Verification items for the finished model (mm, model axes). A direction names the side the tool comes from. Coordinates: 2 decimals unless noted, no trailing zeros. Loops run counter-clockwise (first coordinate to the right, second up) from the corner with the lowest first, then second, coordinate; pieces in that order, holes last. Notation, with made-up numbers: (60, -18) - (71, -18) arc R11 cw to (71, 1) - close; hole circle Ø3 at (-19.5, 88). An arc over 180 degrees is marked (long way). Answer as CSV lines item,"result". Start each with the question number.
1. Set-up check for faces 1 (the flat face through (8.5, 2, 0)), 2 (the cylindrical face through (14.725, 10.143, -36.753)), 3 (the flat face through (19.035, 5.65, 42.465)), 4 (the cylindrical face through (8.292, 4.233, -2.999)): record each of +Z, -Z, +X, -X, +Y, -Y from which the full face is reachable in a straight line by a thin tool's end or side.
2. Cross-section at B-B (x = 20). Enter the section's corners in (y, z), plus the area to 3 significant figures.
3. Release check for a two-part mould opening along Y. For faces 5 (the flat face through (8, 20, 1)), 6 (the flat face through (19, 10, 45)), 7 (the flat face through (15, 10, 17)) record: pulls with the +Y half, pulls with the -Y half, needs draft (parallel to the pull), parting line crosses it, or undercut.
4. Gauge pin test, flat ends, axial feed: P1, Ø10.5, axis at y = 10, z = 0, coming from the +X side; P2, Ø1.5, axis at x = 9, y = 13.5, coming from the -Z side; P3, Ø5.5, axis at x = 18, y = 11, coming from the -Z side. Record the tip position at first contact, or that the pin passes through.
5. Cross-section at D-D (x = 1.75). Enter the section's corners in (y, z).
6. Cross-section at A-A (z = 0). Enter the section's corners in (x, y), plus the area to 3 significant figures.
7. Material ranges on line 1 (Y direction, x = 15.15, z = -40); line 2 (Y direction, x = 0.5, z = 0); line 3 (Z direction, x = 18.25, y = 6.75), recorded low to high. Write a range as [from, to].
8. Cross-section at C-C (y = 18). Enter the section's corners in (x, z).
Autodesk Inventor part; units mm, degrees
ref_plane "YZ Plane" through (0, 0, 0) normal (1, 0, 0) x (0, 1, 0)
ref_plane "XZ Plane" through (0, 0, 0) normal (0, 1, 0) x (-1, 0, 0)
ref_plane "XY Plane" through (0, 0, 0) normal (0, 0, 1) x (1, 0, 0)
sketch "Sketch1" plane through (0, 0, 0) normal (0, 1, 0) x (-1, 0, 0)
  line L0 (0, 0) -> (-20, 0)
  line L1 (-20, 0) -> (-20, -40)
  line L2 (-20, -40) -> (0, 0)
  line L3 (-21.5, -50) -> (-18.5, -50)
  line L4 (-18.5, -50) -> (-18.5, -30)
  line L5 (-18.5, -30) -> (-21.5, -30)
  line L6 (-21.5, -30) -> (-21.5, -50)
  line L7 (-21.5, -50) -> (-18.5, -30) construction
  line L8 (-18.5, -50) -> (-21.5, -30) construction
  line L9 (1.5, 10) -> (-1.5, 10)
  line L10 (-1.5, 10) -> (-1.5, -10)
  line L11 (-1.5, -10) -> (1.5, -10)
  line L12 (1.5, -10) -> (1.5, 10)
  line L13 (1.5, 10) -> (-1.5, -10) construction
  line L14 (-1.5, 10) -> (1.5, -10) construction
  line L15 (-1.5, 10) -> (-21.5, -30)
  line L16 (1.5, -10) -> (-18.5, -50)
  line L17 (1.5, -10) -> (1.5, 10)
  line L18 (1.5, -10) -> (1.5, 10)
  line L19 (1.5, 10) -> (-8.5, 10)
  line L20 (-8.5, 10) -> (-8.5, -10)
  line L21 (-8.5, -10) -> (1.5, -10)
  line L22 (1.5, -10) -> (1.5, 10)
  line L23 (0, 0) -> (10, 0)
  line L24 (0, 0) -> (10, 0) construction
  line L25 (-20, 40) -> (0, 0)
  line L26 (-21.5, 50) -> (-18.5, 50)
  line L27 (-18.5, 50) -> (-18.5, 30)
  line L28 (-18.5, 30) -> (-21.5, 30)
  line L29 (-21.5, 30) -> (-21.5, 50)
  line L30 (-1.5, -10) -> (-1.5, 10)
  line L31 (-1.5, 10) -> (1.5, 10)
  line L32 (-1.5, -10) -> (-21.5, 30)
  line L33 (1.5, 10) -> (-18.5, 50)
  line L34 (1.5, 10) -> (1.5, -10)
  point P0 (-7.3579, -1.7157)
  point P1 (-11.5, -10)
  point P2 (-11.5, -10)
  point P3 (-8.5, -4)
  point P4 (-8.5, 4)
  dimension "d0" = 20
  dimension "d1" = 40
  dimension "d2" = 3
  dimension "d3" = 20
  dimension "d4" = 3
  dimension "d5" = 20
  dimension "d31" = 10
  dimension "d32" = 20
  dimension "d42" = 10
  dimension "d43" = 0
extrude "Extrusion1" add sketch "Sketch1" along normal blind 20 contours L2 L10 L0 | L23 L12 L11 L10 L2 | L25 L10 L9 L12 L23 | L0 L10 L25 | L10 L2 L32 L0 | L0 L15 L25 L10 | L10 L32 L2 | L25 L15 L10 | L15 L20 L0 | L32 L20 L19 L25 L15 | L32 L2 L21 L20 L15 | L0 L20 L32 | L32 L21 L2 | L11 L16 L4 L2 L21 | L9 L19 L25 L27 L33 | L15 L25 L19 | L20 L21 L2 L4 L5 L1 L15 | L32 L28 L27 L25 L19 L20 | L3 L6 L5 L1 L2 L4 | L27 L28 L29 L26 | L1 L5 L15 | L2 L1 L5 L4
sketch "Sketch2" plane through (-1.5, 0, -10) normal (-1, 0, 0) x (0, 0, 1)
  circle A0 centre (10, 10) radius 3
  line L0 (0, 0) -> (20, 0)
  line L1 (20, 0) -> (20, 20)
  point P0 (10, 0)
  dimension "d8" = 6
  dimension "d9" = 10
  dimension "d44" = 10
sketch "Sketch3" plane through (21.5, 0, -30) normal (1, 0, 0) x (0, 0, -1)
  circle A0 centre (10, 10) radius 3.25
  line L0 (0, 20) -> (20, 20)
  line L1 (20, 0) -> (20, 20)
  point P0 (-30, 0)
  dimension "d11" = 6.5
  dimension "d12" = 10
  dimension "d13" = 10
extrude "Extrusion2" cut sketch "Sketch2" against normal through all
extrude "Extrusion3" cut sketch "Sketch3" against normal through all
sketch "Sketch4" plane through (21.5, 0, -30) normal (1, 0, 0) x (0, 0, -1)
  circle A0 centre (10, 10) radius 3.25
  line L0 (10, 15.7735) -> (15, 12.8868)
  line L1 (15, 12.8868) -> (15, 7.1132)
  line L2 (15, 7.1132) -> (10, 4.2265)
  line L3 (10, 4.2265) -> (5, 7.1132)
  line L4 (5, 7.1132) -> (5, 12.8868)
  line L5 (5, 12.8868) -> (10, 15.7735)
  line L6 (20, 0) -> (20, 20)
  point P0 (-30, 0)
  point P1 (10, 10)
  dimension "d19" = 10
extrude "Extrusion4" cut sketch "Sketch4" against normal blind 5
fillet "Fillet2" radius 5 1 edges at (21.5, 10, -30)
mirror "Mirror1" about plane through (0, 0, 0) normal (0, 0, 1) of "Extrusion4", "Extrusion3"
sketch "Sketch7" plane through (8.5, 0, 4) normal (1, 0, 0) x (0, 0, -1)
  circle A0 centre (4, 10) radius 3
  circle A1 centre (4, 10) radius 6.5
  point P0 (4, 0)
  dimension "d52" = 13
extrude "Extrusion6" cut sketch "Sketch7" along normal mid plane 2 contours A0 | A1
fillet "Fillet8" radius 5 2 edges at (-1.5, 10, 10) (-1.5, 10, -10)
fillet "Fillet9" radius 5 2 edges at (18.5, 10, 50) (18.5, 10, -50)
ref_plane "Work Plane1" through (0, 0, 0) normal (0, 0, 1) x (1, 0, 0)
properties part number "Bottom_Foot_Standoff" material "PET Plastic"
Values follow:
1,face 1,"+X, +Y, -Y"
1,face 2,"+X, -X"
1,face 3,"+X"
1,face 4,"none"
2,outline,"(0, -49.74) - (20, -49.74) - (20, -27) - (0, -27) - close; (0, 27) - (20, 27) - (20, 49.74) - (0, 49.74) - close; hole (4.23, -40) - (7.11, -45) - (12.89, -45) - (15.77, -40) - (12.89, -35) - (7.11, -35) - close; hole (4.23, 40) - (7.11, 35) - (12.89, 35) - (15.77, 40) - (12.89, 45) - (7.11, 45) - close"
2,area,"736 mm²"
3,face 5,"pulls with the +Y half"
3,face 6,"undercut"
3,face 7,"needs draft"
4,P1,"stops at x = 7.5"
4,P2,"stops at z = -32.5"
4,P3,"stops at z = -49.93"
5,outline,"(0, -16.5) - (20, -16.5) - (20, 16.5) - (0, 16.5) - close; hole circle Ø6 at (10, 0)"
6,outline,"(-1.5, 0) - (8.5, 0) - (8.5, 3.5) - (7.5, 3.5) - (7.5, 7) - (-1.5, 7) - close; (-1.5, 13) - (7.5, 13) - (7.5, 16.5) - (8.5, 16.5) - (8.5, 20) - (-1.5, 20) - close"
6,area,"133 mm²"
7,line 1,"y = [0, 6.75], [13.25, 20]"
7,line 2,"y = [0, 7], [13, 20]"
7,line 3,"z = [-48.72, -44.37], [-35.63, -23.5], [23.5, 35.63], [44.37, 48.72]"
8,outline,"(-1.5, -8.82) arc R5 ccw to (-0.97, -11.06) - (17.12, -47.24) arc R5 ccw to (21.5, -50) - (21.5, -31.18) arc R5 ccw to (20.97, -28.94) - (8.5, -4) - (8.5, 4) - (21.5, 30) - (21.5, 50) arc R5 ccw to (17.12, 47.24) - (-0.97, 11.06) arc R5 ccw to (-1.5, 8.82) - close"
